from build123d import *

# Parameters (mm, degrees)
F0_W     = 20
F0_H     = 34.5
F1_DEPTH = 6
F2_DEPTH = 20
F3_W     = 5.5
F3_H     = 3.0757111441
F3_W_2   = 0.5
F3_H_2   = 1.4242888559
F4_DEPTH = 50
F5_W     = 8
F5_H     = 3
F6_DEPTH = 50
F7_SIZE  = 2.99999


# Not quite as in the source:
# - a fillet or chamfer is up to 0.001 mm smaller than in the source, because OpenCascade refuses the exact size


with BuildPart() as f1:
    # F0 (on Top) → F1 (new body)
    with BuildSketch(Plane.XY):
        with Locations((10, 17.25)):
            Rectangle(F0_W, F0_H)
    extrude(amount=F1_DEPTH)

    # F2 (add): a face of the model
    f2_faces = [f1.faces().sort_by_distance(p)[0] for p in [
        (20, 17.25, 3),
    ]]
    extrude(f2_faces, amount=F2_DEPTH)

    # F3 (on face) → F4 (cut)
    with BuildSketch(Plane(origin=(0, 0, 0), x_dir=(0, -1, 0), z_dir=(-1, 0, 0))):
        Polygon((-20, 6.5), (-14.5, 6.5), (-14.5, 6), (-14, 6), (-14, 9.0350331739), (-20.5, 9.0350331739), (-20.5, 6), (-20, 6), align=None)
        with Locations((-17.25, 4.4621444279)):
            Rectangle(F3_W, F3_H)
        with Locations((-14.25, 4.4621444279)):
            Rectangle(F3_W_2, F3_H)
        with Locations((-20.25, 4.4621444279)):
            Rectangle(F3_W_2, F3_H)
        with Locations((-17.25, 2.2121444279)):
            Rectangle(F3_W, F3_H_2)
    extrude(amount=-F4_DEPTH, mode=Mode.SUBTRACT)

    # F5 (on face) → F6 (cut)
    with BuildSketch(Plane(origin=(0, 0, 0), x_dir=(0, -1, 0), z_dir=(-1, 0, 0))):
        with Locations((-27.5, 4.5)):
            Rectangle(F5_W, F5_H)
        with Locations((-7, 4.5)):
            Rectangle(F5_W, F5_H)
    extrude(amount=-F6_DEPTH, mode=Mode.SUBTRACT)

    # F7 (size 3 in the source; OpenCascade refuses exactly that, so slightly less here)
    f7_edges = [f1.edges().sort_by_distance(p)[0] for p in [
        (20, 11, 6),
        (20, 3, 6),
        (20, 31.5, 6),
        (20, 23.5, 6),
    ]]
    chamfer(f7_edges, length=F7_SIZE)


solid = f1.part
Can you work these out from the model? Positions are in its coordinate system, mm. A direction names the side the tool comes from. Give positions to 0.01 mm unless a question says otherwise; leave off trailing zeros. Order: outer loops, then holes, each group sorted by start corner. A loop starts at its lowest first (then second) coordinate and runs counter-clockwise, first axis right, second up. Notation, with made-up numbers: M 79.5,17.25 L 106.5,17.25 A16 cw 106.5,44.25 Z; hole C -34,2 d5. An arc over 180 degrees is marked long. One line per item, written item: value.
Item 1: For faces 1 (the face through (20, 17, 1.5)), 2 (the face through (40, 17, 1)), which set-ups out of +Z, -Z, +X, -X, +Y, -Y let a thin tool reach every point of the face, with its end or its side?
Verdict:
face 1: +Z, +X, -X
face 2: +Z, -Z, +X, +Y, -Y
Item 2: If we section it at C-C on y = 10: Write out the boundary of the cut face in (x, z), and give its area (3 significant figures).
Verdict:
outline: M 0,0 L 40,0 L 40,3 L 0,3 Z
area: 120 mm2
Item 3: If we section it at D-D on z = 4: Write out the boundary of the cut face in (x, y).
Verdict:
outline: M 0,0 L 40,0 L 40,2 L 0,2 Z; M 0,12 L 40,12 L 40,14 L 0,14 Z; M 0,20.5 L 40,20.5 L 40,22.5 L 0,22.5 Z; M 0,32.5 L 40,32.5 L 40,34.5 L 0,34.5 Z
Item 4: If we mould it in two halves opening along Y, with no side actions, what happens to faces 3 (the face through (20, 20.5, 4)), 4 (the face through (20, 0, 3)), 5 (the face through (0, 17, 1))? For each: pulls with the +Y half, pulls with the -Y half, needs draft (parallel to the pull), parting line crosses it, or undercut.
Verdict:
face 3: undercut
face 4: pulls with the -Y half
face 5: needs draft
Item 5: For pin 1 (6.5 mm diameter, centred on x = 18.5, y = 8.5, fed in from +Z); pin 2 (1.5 mm diameter, centred on x = 15, z = 4, fed in from -Y); pin 3 (9 mm diameter, centred on x = 14, y = 27, fed in from +Z); pin 4 (1 mm diameter, centred on x = 23.5, y = 12.5, fed in from +Z), each with a flat end and sliding along its axis, tell me the tip position at first contact or that it passes through.
Verdict:
pin 1: z = 3.75
pin 2: y = 0
pin 3: z = 4
pin 4: z = 5
Item 6: Please list where these lines run through material, in increasing order: line 1 (Y direction, x = 37.5, z = 4.75); line 2 (Y direction, x = 9.5, z = 3.5); line 3 (Y direction, x = 4, z = 2.5).
Verdict:
line 1: 0 to 1.25, 12.75 to 14, 20.5 to 21.75, 33.25 to 34.5
line 2: 0 to 2.5, 11.5 to 14, 20.5 to 23, 32 to 34.5
line 3: 0 to 14.5, 20 to 34.5
Item 7: If we section it at A-A on z = 2: Write out the boundary of the cut face in (x, y), and give its area (3 significant figures).
Verdict:
outline: M 0,0 L 40,0 L 40,14.5 L 0,14.5 Z; M 0,20 L 40,20 L 40,34.5 L 0,34.5 Z
area: 1,160 mm2
